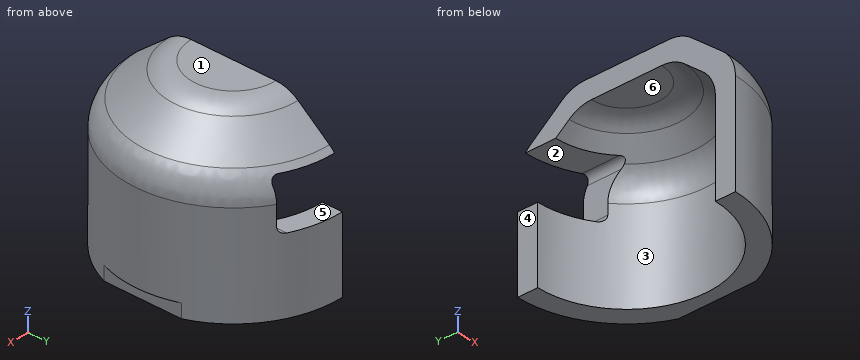
Autodesk Inventor part; units mm, degrees
ref_plane "РабПлоскость1" through (7, 16.35, -7.7) normal (0, 1, 0) x (-1, 0, 0)
ref_plane "YZ Plane" through (0, 0, 0) normal (1, 0, 0) x (0, 1, 0)
ref_plane "XZ Plane" through (0, 0, 0) normal (0, 1, 0) x (-1, 0, 0)
sketch "Эскиз1" plane through (0, 0, 0) normal (1, 0, 0) x (0, 1, 0)
  line L0 (0, 1) -> (-7.8216, 1)
  line L1 (-7.8216, 1) -> (-7.8216, 3.85)
  line L2 (-7.8216, 3.85) -> (0, 3.85)
  line L3 (0, 3.85) -> (0, 1)
  line L4 (-15.5, -46.55) -> (-15.5, -19.55)
  line L5 (-15.5, -19.55) -> (-12.65, -19.55)
  line L6 (-12.65, -19.55) -> (-12.65, -2.466)
  line L7 (-12.65, -2.466) -> (-15.5, -2.466)
  line L8 (-15.5, -2.466) -> (-15.5, -19.55)
  line L9 (-12.15, -9.434) -> (-12.15, -39.916)
  line L10 (-15.5, -2.466) -> (-7.8216, 3.85)
  line L11 (-7.8216, 3.85) -> (-6.0111, 1.649)
  line L12 (-6.0111, 1.649) -> (-13.6895, -4.6671)
  line L13 (-13.6895, -4.6671) -> (-15.5, -2.466)
  line L14 (-6.8, -2) -> (-6.8, -7.7)
  line L15 (0, -56.63) -> (0, 13.93)
  point P0 (0, 0)
  point P1 (-6.8, 1)
  point P2 (-12.65, -3.812)
  dimension "d0" = 0.5
  dimension "d1" = 2.85
  dimension "d2" = 2.85
  dimension "d3" = 50.56
  dimension "d4" = 0
  dimension "d5" = 1
  dimension "d6" = 2.85
  dimension "d7" = 0
revolve "Вращение1" add sketch "Эскиз1" angle 180 about axis through (0, 0, -10) along (0, 0, 1)
ref_plane "РабПлоскость1" through (7, 16.35, -7.7) normal (0, 1, 0) x (-1, 0, 0)
sketch "Эскиз2" plane through (7, 16.35, -7.7) normal (0, 1, 0) x (-1, 0, 0)
  line L0 (0, 0) -> (14, 0)
  line L1 (14, 0) -> (14, 5)
  line L2 (0, 5) -> (14, 5)
  line L3 (0, 0) -> (0, 5)
  line L4 (0, -1) -> (14, -1)
  line L5 (15, 0) -> (15, 5)
  line L6 (14, 6) -> (0, 6)
  line L7 (-1, 5) -> (-1, 0)
  arc A0 (-1, 0) -> (0, -1) centre (0, 0) ccw
  arc A1 (0, 6) -> (-1, 5) centre (0, 5) ccw
  arc A2 (15, 5) -> (14, 6) centre (14, 5) ccw
  arc A3 (14, -1) -> (15, 0) centre (14, 0) ccw
  point P0 (7, 7.7)
  dimension "d9" = 1
  dimension "d10" = 1
  dimension "d11" = 1
  dimension "d12" = 1
  dimension "d13" = 1
  dimension "d14" = 1
extrude "Выдавливание1" cut sketch "Эскиз2" against normal blind 10 contours L3 L2 L1 L0 | A0 L7 A1 L6 A2 L5 A3 L4
fillet "Сопряжение1" radius 5 4 edges at (7.8216, 0, 3.85) (14.938, -4.1361, -2.466) (6.8, 0, 1) (11.916, -4.2464, -3.812)
sketch "Эскиз3" plane through (0, -15.5, -19.55) normal (0, 0, -1) x (-1, 0, 0)
  line L0 (-14.4918, 10.0011) -> (-14.4918, 20.9989)
  arc A0 (-14.4918, 20.9989) -> (-14.4918, 10.0011) centre (0, 15.5) ccw
  point P0 (0, 15.5)
extrude "Выдавливание2" cut sketch "Эскиз3" against normal blind 2
properties part number "EncCoverHalf" material "Пластик ПАЭК"
Source: CAD feature listing. Evaluate the final solid. Frame: model axes, mm. Face numbers are marked on the shaded views. A direction names the side the tool comes from. Round coordinates to 2 decimals unless told otherwise and drop trailing zeros. Order: outer loops, then holes, each group sorted by start corner. A loop starts at its lowest first (then second) coordinate and runs counter-clockwise, first axis right, second up. Notation, with made-up numbers: (81, -18.5) -> (124, -18.5) arc R21 cw to (124, -14.5) -> close; hole circle Ø6 at (74, -3). An arc over 180 degrees is marked (long way). One line per item, written item: value. Start each with the question number.
Q1. Draft query along Z for the marked faces 4, 5 and 6. Return one class per face: pulls with the +Z half, pulls with the -Z half, needs draft (parallel to the pull), parting line crosses it, or undercut.
Q2. Material intervals for probe 1 along Y at (x, z) = (2.5, -13.75); probe 2 along Y at (x, z) = (9.75, -5.5); probe 3 along Z at (x, y) = (1, 2.5), sorted ascending.
Q3. Access query for the marked faces 1, 2 and 3. Directions: +Z, -Z, +X, -X, +Y, -Y. A direction counts if a zero-diameter tool reaches every point of the face in a straight line with its end or side. Return the directions, or none.
Q4. Pin query (flat end, axial travel): pin 1 (3 mm diameter, centred on x = 14, y = -4.5, fed in from +Z); pin 2 (1 mm diameter, centred on x = 5, y = 6.5, fed in from -Z); pin 3 (6 mm diameter, centred on x = 3.5, z = -4.5, fed in from -Y); pin 4 (4 mm diameter, centred on x = 4.5, y = -5.5, fed in from +Z). Return the tip coordinate at first contact, or that it passes through.
Q5. Section query A-A (z = -17). Return the cut outline in (x, y), plus the area to 3 significant figures.
Findings below:
1. face 4: needs draft
1. face 5: undercut
1. face 6: pulls with the -Z half
2. probe 1: -15.3 to -12.4, 12.4 to 15.3
2. probe 2: -12.05 to -7.99, 7.99 to 12.05
2. probe 3: 1 to 3.85
3. face 1: +Z, +X, -X, +Y, -Y
3. face 2: -X, +Y
3. face 3: -Z, -X
4. pin 1: z = -0.58
4. pin 2: z = -0.56
4. pin 3: y = -15.49
4. pin 4: z = 3.85
5. outline: (0, -15.5) arc R15.5 ccw to (0, 15.5) -> (0, 12.65) arc R12.65 cw to (0, -12.65) -> close
5. area: 126 mm²
